```python
from build123d import *

# Parameters (mm, degrees)
SKETCH1_R                = 2
BOSS_EXTRUDE1_DEPTH      = 6.5
BOSS_EXTRUDE1_DEPTH_BACK = 2.5
BOSS_EXTRUDE3_DEPTH      = 2.5
FILLET2_R                = 10
SKETCH2_W                = 47
SKETCH2_H                = 5.65
BOSS_EXTRUDE4_DEPTH      = 40.25
SKETCH2_4_W              = 5.4
SKETCH2_4_H              = 11.5
BOSS_EXTRUDE5_DEPTH      = 37
SKETCH2_5_W              = 5.4
SKETCH2_5_H              = 47.5
BOSS_EXTRUDE6_DEPTH      = 37
BOSS_EXTRUDE6_DEPTH_BACK = 6.5
SKETCH4_R                = 4
CUT_EXTRUDE1_DEPTH       = 2.4
SKETCH5_R                = 1.75
CUT_EXTRUDE2_DEPTH       = 36.2
SKETCH5_4_R              = 1.75
CUT_EXTRUDE3_DEPTH       = 12
SKETCH5_5_R              = 1.75
BOSS_EXTRUDE7_DEPTH      = 5.65
LPATTERN2_COUNT          = 2
LPATTERN2_PITCH          = 28.7
MIRROR1_COPY_1_SKETCH_R  = 1.75
MIRROR1_COPY_1_DEPTH     = 36.2
MIRROR1_COPY_2_SKETCH_R  = 1.75
MIRROR1_COPY_2_DEPTH     = 12
MIRROR1_COPY_3_SKETCH_R  = 1.75
MIRROR1_COPY_3_DEPTH     = 5.65
MIRROR1_COPY_4_SKETCH_R  = 1.75
MIRROR1_COPY_4_DEPTH     = 36.2
SKETCH7_R                = 10.5
CUT_EXTRUDE4_DEPTH       = 5.65
FILLET3_R                = 10
FILLET5_R                = 5
FILLET6_R                = 5
FILLET12_R               = 5
CUT_EXTRUDE5_DEPTH       = 69
CUT_EXTRUDE7_DEPTH       = 40


with BuildPart() as part:
    # Sketch1 → Boss-Extrude1 (new body, two sides)
    with BuildSketch(Plane.XY) as boss_extrude1_sk:
        with BuildLine():
            ThreePointArc((7.5, -13.5), (0, -6), (-7.5, -13.5))
            Line((-7.5, -13.5), (-7.5, -20))
            Line((-7.5, -20), (-34, -20))
            Line((-34, -20), (-34, 20))
            Line((-34, 20), (-14.186260959, 20))
            ThreePointArc((-14.186260959, 20), (0, 31.5), (14.186260959, 20))
            Line((14.186260959, 20), (34, 20))
            Line((34, 20), (34, -20))
            Line((34, -20), (7.5, -20))
            Line((7.5, -20), (7.5, -13.5))
        make_face()
        with Locations((16, 11)):
            Circle(SKETCH1_R, mode=Mode.SUBTRACT)
        with Locations((-16, 11)):
            Circle(SKETCH1_R, mode=Mode.SUBTRACT)
        with Locations((16, -13.7)):
            Circle(SKETCH1_R, mode=Mode.SUBTRACT)
        with Locations((-16, -13.7)):
            Circle(SKETCH1_R, mode=Mode.SUBTRACT)
        with BuildLine():
            ThreePointArc((-5.3, 15.5), (0, 10.2), (5.3, 15.5))
            Line((5.3, 15.5), (5.3, 18.5))
            ThreePointArc((5.3, 18.5), (0, 23.8), (-5.3, 18.5))
            Line((-5.3, 18.5), (-5.3, 15.5))
        make_face(mode=Mode.SUBTRACT)
    extrude(amount=BOSS_EXTRUDE1_DEPTH)
    extrude(boss_extrude1_sk.sketch, amount=-BOSS_EXTRUDE1_DEPTH_BACK)

    # Sketch1<5> → Boss-Extrude3 (add)
    with BuildSketch(Plane.XY):
        Polygon((-34, -67.5), (-26.6, -67.5), (-7.5, -20), (-34, -20), align=None)
    extrude(amount=-BOSS_EXTRUDE3_DEPTH)

    # Fillet2
    fillet2_edges = [part.edges().sort_by_distance(p)[0] for p in [
        (-34, 20, 2),
        (34, 20, 2),
        (34, -20, 2),
    ]]
    fillet(fillet2_edges, radius=FILLET2_R)

    # Sketch2 → Boss-Extrude4 (add)
    with BuildSketch(Plane.XY.offset(6.5)):
        with Locations((-0.1, -0.875)):
            Rectangle(SKETCH2_W, SKETCH2_H)
        with BuildLine():
            Line((-23.6, 1.95), (23.4, 1.95))
            ThreePointArc((23.4, 1.95), (13.763613768, 8.149784472), (2.641305414, 10.905056506))
            ThreePointArc((2.641305414, 10.905056506), (-0.013421952, 10.200016995), (-2.664544331, 10.918493315))
            ThreePointArc((-2.664544331, 10.918493315), (-13.88218364, 8.184790241), (-23.6, 1.95))
        make_face()
    extrude(amount=BOSS_EXTRUDE4_DEPTH)

    # Sketch2<4> → Boss-Extrude5 (add)
    with BuildSketch(Plane.XY.offset(6.5)):
        with BuildLine():
            ThreePointArc((-23.6, -3.7), (-27.066660678, -5.093061794), (-28.6, -8.5))
            Line((-28.6, -8.5), (-34, -8.5))
            ThreePointArc((-34, -8.5), (-30.956929628, -1.12839061), (-23.6, 1.95))
            Line((-23.6, 1.95), (-23.6, -3.7))
        make_face()
        with Locations((-31.3, -14.25)):
            Rectangle(SKETCH2_4_W, SKETCH2_4_H)
    extrude(amount=BOSS_EXTRUDE5_DEPTH)

    # Sketch2<5> → Boss-Extrude6 (add, two sides)
    with BuildSketch(Plane.XY.offset(6.5)) as boss_extrude6_sk:
        with Locations((-31.3, -43.75)):
            Rectangle(SKETCH2_5_W, SKETCH2_5_H)
    extrude(amount=BOSS_EXTRUDE6_DEPTH)
    extrude(boss_extrude6_sk.sketch, amount=-BOSS_EXTRUDE6_DEPTH_BACK)

    # Sketch4 → Cut-Extrude1 (cut)
    with BuildSketch(Plane.XY.offset(6.5)):
        with Locations((-16, 11)):
            Circle(SKETCH4_R)
        with Locations((16, 11)):
            Circle(SKETCH4_R)
        with Locations((16, -13.7)):
            Circle(SKETCH4_R)
        with Locations((-16, -13.7)):
            Circle(SKETCH4_R)
    extrude(amount=-CUT_EXTRUDE1_DEPTH, mode=Mode.SUBTRACT)

    # Sketch5 → Cut-Extrude2 (cut, through all)
    with BuildSketch(Plane(origin=(0, -3.7, 0), x_dir=(-1, 0, 0), z_dir=(0, -1, 0))):
        with Locations((17.6, -12.531088913)):
            Circle(SKETCH5_R)
    cut_extrude2 = extrude(amount=-CUT_EXTRUDE2_DEPTH, mode=Mode.SUBTRACT)

    # Sketch5<4> → Cut-Extrude3 (cut)
    with BuildSketch(Plane(origin=(0, -3.7, 0), x_dir=(-1, 0, 0), z_dir=(0, -1, 0))):
        Polygon((15.85, -15.562177826), (19.35, -15.562177826), (21.1, -12.531088913), (19.35, -9.5), (15.85, -9.5), (14.1, -12.531088913), align=None)
        with Locations((17.6, -12.531088913)):
            Circle(SKETCH5_4_R, mode=Mode.SUBTRACT)
    cut_extrude3 = extrude(amount=-CUT_EXTRUDE3_DEPTH, mode=Mode.SUBTRACT)

    # Sketch5<5> → Boss-Extrude7 (add)
    with BuildSketch(Plane(origin=(0, -3.7, 0), x_dir=(-1, 0, 0), z_dir=(0, -1, 0))):
        Polygon((15.85, -15.562177826), (19.35, -15.562177826), (21.1, -12.531088913), (19.35, -9.5), (15.85, -9.5), (14.1, -12.531088913), align=None)
        with Locations((17.6, -12.531088913)):
            Circle(SKETCH5_5_R, mode=Mode.SUBTRACT)
    boss_extrude7 = extrude(amount=-BOSS_EXTRUDE7_DEPTH)

    # LPattern2: Cut-Extrude2, Cut-Extrude3, Boss-Extrude7 ×2
    with Locations(*[(0, 0, i * LPATTERN2_PITCH) for i in range(1, LPATTERN2_COUNT)]):
        add(cut_extrude2, mode=Mode.SUBTRACT)
        add(cut_extrude3, mode=Mode.SUBTRACT)
        add(boss_extrude7)

    # Mirror1: Cut-Extrude3, Boss-Extrude7 across plane
    add(cut_extrude3.mirror(Plane.ZY.offset(0.1)), mode=Mode.SUBTRACT)
    add(boss_extrude7.mirror(Plane.ZY.offset(0.1)))

    # Mirror1 copy 1 sketch → Mirror1 copy 1 (cut, through all)
    with BuildSketch(Plane(origin=(-0.2, -3.7, 28.7), x_dir=(1, 0, 0), z_dir=(0, -1, 0))):
        with Locations((17.6, 12.531088913)):
            Circle(MIRROR1_COPY_1_SKETCH_R)
    extrude(amount=-MIRROR1_COPY_1_DEPTH, mode=Mode.SUBTRACT)

    # Mirror1 copy 2 sketch → Mirror1 copy 2 (cut)
    with BuildSketch(Plane(origin=(-0.2, -3.7, 28.7), x_dir=(1, 0, 0), z_dir=(0, -1, 0))):
        Polygon((15.85, 15.562177826), (19.35, 15.562177826), (21.1, 12.531088913), (19.35, 9.5), (15.85, 9.5), (14.1, 12.531088913), align=None)
        with Locations((17.6, 12.531088913)):
            Circle(MIRROR1_COPY_2_SKETCH_R, mode=Mode.SUBTRACT)
    extrude(amount=-MIRROR1_COPY_2_DEPTH, mode=Mode.SUBTRACT)

    # Mirror1 copy 3 sketch → Mirror1 copy 3 (add)
    with BuildSketch(Plane(origin=(-0.2, -3.7, 28.7), x_dir=(1, 0, 0), z_dir=(0, -1, 0))):
        Polygon((15.85, 15.562177826), (19.35, 15.562177826), (21.1, 12.531088913), (19.35, 9.5), (15.85, 9.5), (14.1, 12.531088913), align=None)
        with Locations((17.6, 12.531088913)):
            Circle(MIRROR1_COPY_3_SKETCH_R, mode=Mode.SUBTRACT)
    extrude(amount=-MIRROR1_COPY_3_DEPTH)

    # Mirror1 copy 4 sketch → Mirror1 copy 4 (cut, through all)
    with BuildSketch(Plane(origin=(-0.2, -3.7, 0), x_dir=(1, 0, 0), z_dir=(0, -1, 0))):
        with Locations((17.6, 12.531088913)):
            Circle(MIRROR1_COPY_4_SKETCH_R)
    extrude(amount=-MIRROR1_COPY_4_DEPTH, mode=Mode.SUBTRACT)

    # Sketch7 → Cut-Extrude4 (cut)
    with BuildSketch(Plane.ZY.offset(34)):
        with BuildLine():
            ThreePointArc((28.34667488, -42.854044185), (28.835378228, -44.647985724), (29, -46.5))
            ThreePointArc((29, -46.5), (24.341660723, -55.224964183), (14.5, -56.208243919))
            ThreePointArc((14.5, -56.208243919), (15.43971668, -63.273798399), (9.7, -67.5))
            Line((9.7, -67.5), (43.5, -67.5))
            Line((43.5, -67.5), (43.5, -32.5))
            ThreePointArc((43.5, -32.5), (37.856610976, -40.506401793), (28.34667488, -42.854044185))
        make_face()
        with Locations((18.5, -46.5)):
            Circle(SKETCH7_R)
    extrude(amount=-CUT_EXTRUDE4_DEPTH, mode=Mode.SUBTRACT)

    # Fillet3
    fillet3_edges = [part.edges().sort_by_distance(p)[0] for p in [
        (-31.3, -42.854044185, 28.34667488),
    ]]
    fillet(fillet3_edges, radius=FILLET3_R)

    # Fillet5
    fillet5_edges = [part.edges().sort_by_distance(p)[0] for p in [
        (-31.3, -56.208243919, 14.5),
    ]]
    fillet(fillet5_edges, radius=FILLET5_R)

    # Fillet6
    fillet6_edges = [part.edges().sort_by_distance(p)[0] for p in [
        (7.5, -20, 2),
    ]]
    fillet(fillet6_edges, radius=FILLET6_R)

    # Fillet12
    fillet12_edges = [part.edges().sort_by_distance(p)[0] for p in [
        (-7.5, -20, 3.25),
    ]]
    fillet(fillet12_edges, radius=FILLET12_R)

    # Sketch10 → Cut-Extrude5 (cut, through all)
    with BuildSketch(Plane.ZY.offset(34)):
        with BuildLine():
            Line((6.88909431, -26.942221984), (9.812269185, -29.672615481))
            ThreePointArc((9.812269185, -29.672615481), (9.896611038, -32.146051644), (7.423174875, -32.230393497))
            Line((7.423174875, -32.230393497), (4.5, -29.5))
            ThreePointArc((4.5, -29.5), (4.415658147, -27.026563837), (6.88909431, -26.942221984))
        make_face()
        with BuildLine():
            Line((35.211828487, -29.423174875), (37.942221984, -26.5))
            ThreePointArc((37.942221984, -26.5), (40.415658147, -26.415658147), (40.5, -28.88909431))
            Line((40.5, -28.88909431), (37.769606503, -31.812269185))
            ThreePointArc((37.769606503, -31.812269185), (35.29617034, -31.896611038), (35.211828487, -29.423174875))
        make_face()
        with BuildLine():
            Line((9.788171513, -60.576825125), (7.057778016, -63.5))
            ThreePointArc((7.057778016, -63.5), (4.584341853, -63.584341853), (4.5, -61.11090569))
            Line((4.5, -61.11090569), (7.230393497, -58.187730815))
            ThreePointArc((7.230393497, -58.187730815), (9.70382966, -58.103388962), (9.788171513, -60.576825125))
        make_face()
    extrude(amount=-CUT_EXTRUDE5_DEPTH, mode=Mode.SUBTRACT)

    # Sketch11 → Cut-Extrude7 (cut)
    with BuildSketch(Plane(origin=(0, 20, 0), x_dir=(1, 0, 0), z_dir=(0, 1, 0))):
        Polygon((29.466805248, 2.5), (26.75, -1.38), (22.96, -1.38), (20.243194752, 2.5), align=None)
        Polygon((-20.443194752, 2.5), (-29.666805248, 2.5), (-26.95, -1.38), (-23.16, -1.38), align=None)
    extrude(amount=-CUT_EXTRUDE7_DEPTH, mode=Mode.SUBTRACT)


solid = part.part
```
Verification items for the finished model (mm, model axes). A direction names the side the tool comes from. Coordinates: 2 decimals unless noted, no trailing zeros. Order: outer loops, then holes, each group sorted by start corner. A loop starts at its lowest first (then second) coordinate and runs counter-clockwise, first axis right, second up. Notation, with made-up numbers: (2, 20.25) - (43, 20.25) arc R27 cw to (43, 52.25) - close; hole circle Ø8 at (-26, 33). An arc over 180 degrees is marked (long way). Return JSON: item names as keys, results as strings.
(1) Go/stop test with flat-tipped pins: pin 1 (2.5 mm diameter, centred on x = 20.5, z = 0.5, fed in from +Y); pin 2 (5 mm diameter, centred on x = -19, z = 41, fed in from +Y); pin 3 (10 mm diameter, centred on x = -18, z = 39, fed in from -Y). Record where each tip stops, or that it passes through.
Filled sheet:
{"pin 1": "stops at y = 20", "pin 2": "stops at y = 5.1", "pin 3": "stops at y = -3.7"}
(2) Mould release check, pull along Z, two halves, no side actions. Record for faces 1 (the flat face through (-25, 0, 1.38)), 2 (the cylindrical face through (-31.3, -26.4, 40.4)), 3 (the flat face through (-30, -15, 43.5)), 4 (the flat face through (-19, 20, 2)): pulls with the +Z half, pulls with the -Z half, needs draft (parallel to the pull), parting line crosses it, or undercut.
Filled sheet:
{"face 1": "pulls with the -Z half", "face 2": "undercut", "face 3": "pulls with the +Z half", "face 4": "needs draft"}
(3) Thickness scan on line 1 along Y through (x, z) = (16, 0); line 2 along Y through (x, z) = (-16, 5); line 3 along X through (y, z) = (-1, 41). Record the ranges inside material, lowest first.
Filled sheet:
{"line 1": "y = -20 to -15.7, -11.7 to 9, 13 to 20", "line 2": "y = -20 to -17.7, -9.7 to 7, 15 to 20", "line 3": "x = -30.83 to -19.33, -15.87 to 15.67, 19.13 to 23.4"}
(4) Access from +Z, -Z, +X, -X, +Y, -Y to the whole of each face (thin tool, end or side, straight path). Record for faces 5 (the cylindrical face through (-13.73, 8.25, 26.34)), 6 (the cylindrical face through (0.1, 23.8, 2.1)), 7 (the flat face through (-7.5, -14.5, 0.1)), 8 (the flat face through (-19, 1.95, 11)).
Filled sheet:
{"face 5": "+Z, -X, +Y", "face 6": "+Z, -Z", "face 7": "+Z, -Z, -Y", "face 8": "+Y"}
(5) Section check A-A, the plane z = 18.5. Record the cut outline in (x, y).
Filled sheet:
{"outline": "(-34, -36) - (-28.6, -36) - (-28.6, -8.5) arc R5 cw to (-23.6, -3.7) - (23.4, -3.7) - (23.4, 1.95) arc R35 ccw to (2.64, 10.91) arc R5.3 cw to (-2.66, 10.92) arc R35 ccw to (-23.6, 1.95) arc R10.45 ccw to (-34, -8.5) - close"}
(6) Section check B-B, the plane y = -52. Record the cut outline in (x, z), and give its area (3 significant figures).
Filled sheet:
{"outline": "(-34, -2.5) - (-20.37, -2.5) - (-20.37, 0) - (-28.6, 0) - (-28.6, 9.56) - (-34, 9.56) - close", "area": "85.7 mm^2"}
